from build123d import *

# Parameters (mm, degrees)
SKETCH1_R           = 12.7
SKETCH1_R_2         = 4.7625
BOSS_EXTRUDE1_DEPTH = 9.525
FILLET1_R           = 6.35
FILLET2_R           = 3.175
CHAMFER1_SIZE       = 1.5875


with BuildPart() as part:
    # Sketch1 → Boss-Extrude1 (new body)
    # profile 1 of 2: a face of its own
    with BuildSketch(Plane.XY):
        with BuildLine():
            Line((165.1, 12.7), (0, 12.7))
            ThreePointArc((0, 12.7), (8.980256121, 8.980256121), (12.7, 0))
            ThreePointArc((12.7, 0), (8.980256121, -8.980256121), (0, -12.7))
            Line((0, -12.7), (44.45, -12.7))
            Line((44.45, -12.7), (88.9, -31.75))
            Line((88.9, -31.75), (101.6, -31.75))
            ThreePointArc((101.6, -31.75), (127, -6.35), (152.4, -31.75))
            Line((152.4, -31.75), (165.1, -31.75))
            Line((165.1, -31.75), (165.1, 12.7))
        make_face()
    # profile 2 of 2: a face of its own
    with BuildSketch(Plane.XY):
        Circle(SKETCH1_R)
        with Locations(Location((0, 0, 0), (0, 0, 180))):
            Circle(SKETCH1_R_2, mode=Mode.SUBTRACT)
    extrude(amount=BOSS_EXTRUDE1_DEPTH)

    # Fillet1
    fillet1_edges = [part.edges().sort_by_distance(p)[0] for p in [
        (165.1, 12.7, 4.7625),
        (165.1, -31.75, 4.7625),
    ]]
    fillet(fillet1_edges, radius=FILLET1_R)

    # Fillet2
    fillet2_edges = [part.edges().sort_by_distance(p)[0] for p in [
        (101.6, -31.75, 4.7625),
        (152.4, -31.75, 4.7625),
    ]]
    fillet(fillet2_edges, radius=FILLET2_R)

    # Chamfer1
    chamfer1_edges = [part.edges().sort_by_distance(p)[0] for p in [
        (93.750968343, -31.75, 0),
        (66.675, -22.225, 0),
        (22.225, -12.7, 0),
        (-12.7, 0, 0),
        (79.375, 12.7, 0),
        (79.375, 12.7, 9.525),
        (-12.7, 0, 9.525),
        (22.225, -12.7, 9.525),
        (66.675, -22.225, 9.525),
        (165.1, -9.525, 0),
        (165.1, -9.525, 9.525),
        (157.074031657, -31.75, 0),
        (163.240128061, 10.840128061, 0),
        (93.750968343, -31.75, 9.525),
        (163.240128061, -29.890128061, 0),
        (157.074031657, -31.75, 9.525),
        (163.240128061, 10.840128061, 9.525),
        (163.240128061, -29.890128061, 9.525),
        (4.7625, 0, 9.525),
        (127, -6.35, 0),
        (100.718603352, -30.941505276, 0),
        (153.281396648, -30.941505276, 0),
        (127, -6.35, 9.525),
        (100.718603352, -30.941505276, 9.525),
        (153.281396648, -30.941505276, 9.525),
        (4.7625, 0, 0),
    ]]
    chamfer(chamfer1_edges, length=CHAMFER1_SIZE)


solid = part.part
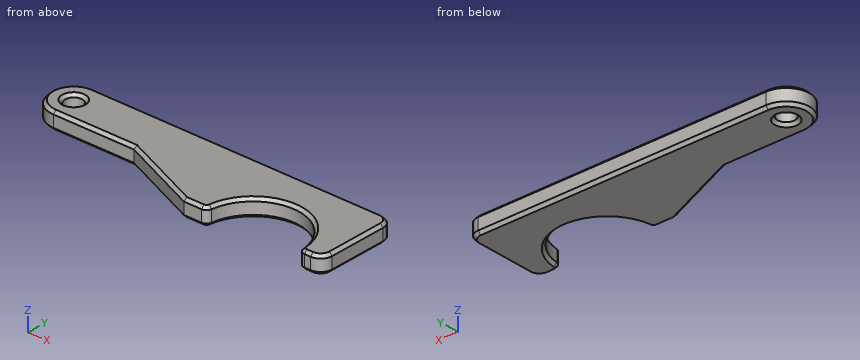
Verification items for the finished model (mm, model axes). Give positions to 0.01 mm unless a question says otherwise; leave off trailing zeros. Write each loop counter-clockwise with the first axis right and the second up, starting at its lowest first coordinate (ties: lowest second). Pieces come first, ordered by that corner, then holes. Notation, with made-up numbers: M 63.5,47.25 L 113.5,47.25 A24 ccw 113.5,79.25 Z; hole C -7,13.5 d5. An arc over 180 degrees is marked long. Use CSV: the item, a comma, the result in double quotes.
1) Cross-section at D-D (x = 55.5). Enter the section's corners in (y, z) (1 decimal).
Final values:
outline,"M -17.4,1.6 L -15.7,0 L 11.1,0 L 12.7,1.6 L 12.7,7.9 L 11.1,9.5 L -15.7,9.5 L -17.4,7.9 Z"
2) Cross-section at C-C (x = 12). Enter the section's corners in (y, z) (1 decimal), plus the area to 3 significant figures.
Final values:
outline,"M -12.7,1.6 L -11.1,0 L 11.1,0 L 12.7,1.6 L 12.7,7.9 L 11.1,9.5 L -11.1,9.5 L -12.7,7.9 Z"
area,"237 mm²"
3) Material ranges on line 1 along Y through (x, z) = (0, 3); line 2 along X through (y, z) = (-0.5, 6.25); line 3 along X through (y, z) = (-24, 6.5), recorded low to high.
Final values:
line 1,"-12.7 to -4.76, 4.76 to 12.7"
line 2,"-12.69 to -4.74, 4.74 to 165.1"
line 3,"70.82 to 102.81, 151.19 to 165.1"
4) Go/stop test with flat-tipped pins: pin 1 Ø12.5 at (x, y) = (0, 0) entering from +Z (3 decimals); pin 2 Ø1 at (y, z) = (-6, 8.5) entering from +X. Record where each tip stops, or that it passes through.
Final values:
pin 1,"z = 9.425"
pin 2,"x = 165.04"
